Print and shaded views of the part. All mm, measured from the part's lowest x, y and z. A direction names the side the tool comes from. Round coordinates to 2 decimals unless told otherwise and drop trailing zeros. Write each loop counter-clockwise with the first axis right and the second up, starting at its lowest first coordinate (ties: lowest second). Pieces come first, ordered by that corner, then holes. Notation, with made-up numbers: (58, 63) -> (62, 63) arc R24 ccw to (62, 94) -> close; hole circle Ø9 at (-39.75, 72.5). An arc over 180 degrees is marked (long way). Use CSV: the item, a comma, the result in double quotes. Start each with the question number.
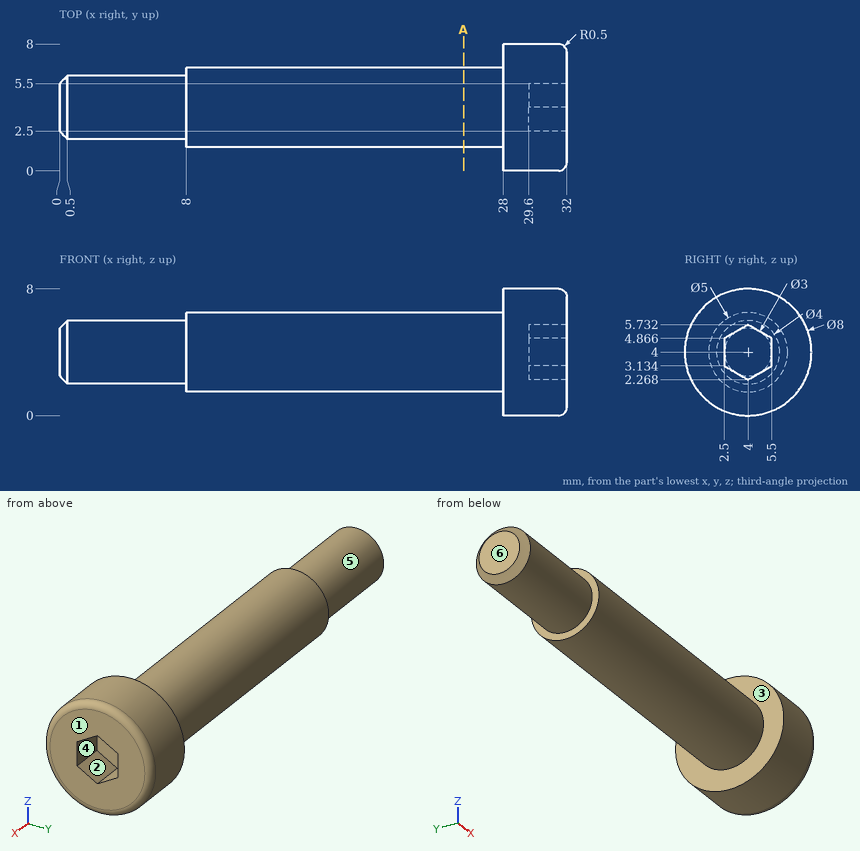
1. Drill centre lines: line 1 along X through (y, z) = (7.25, 5.5); line 2 along Y through (x, z) = (18, 6); line 3 along X through (y, z) = (5, 2). Where is each one in solid material? Low to high. Write a range as [from, to].
2. Flat gauge pins, fed straight in: pin 1 (3 mm diameter, centred on x = 24.5, z = 5, fed in from -Y); pin 2 (3 mm diameter, centred on x = 11.5, y = 4, fed in from -Z). Where does each tip first touch, or does it go through?
3. Band-saw the part on A-A (x = 25.5). List the corners of the cut face in (y, z).
4. Which spindle directions (+Z, -Z, +X, -X, +Y, -Y) get a long thin tool onto all of the face, cutting with end or side? Do the marked faces 1, 2 and 3. Say none if no direction does.
5. Pull direction Y, two halves, no side cores. Call the marked faces 4, 5 and 6: released by +Y, released by -Y, zero draft, split by the parting line, or undercut.
Answers below:
1,line 1,"x = [28, 31.99]"
1,line 2,"y = [2.5, 5.5]"
1,line 3,"x = [8, 32]"
2,pin 1,"stops at y = 1.5"
2,pin 2,"stops at z = 1.5"
3,outline,"circle Ø5 at (4, 4)"
4,face 1,"+Z, -Z, +X, +Y, -Y"
4,face 2,"+X"
4,face 3,"-X"
5,face 4,"undercut"
5,face 5,"split by the parting line"
5,face 6,"zero draft"
